Here's how the part is built. I have some questions about the finished solid (model axes, mm). Face numbers are marked on the shaded views. A direction names the side the tool comes from. Coordinates: 2 decimals unless noted, no trailing zeros.
Item 1: I'm going to push flat-ended pins straight in: pin 1 Ø8 at (x, z) = (43.5, 32.5) entering from -Y; pin 2 Ø15 at (x, z) = (70, 6) entering from -Y; pin 3 Ø21.5 at (x, z) = (-11.5, 15) entering from -Y. Where does each tip first touch, or does it pass through?
Item 2: If I drill on line 1 (X direction, y = -20.5, z = -4.5); line 2 (X direction, y = -19.5, z = 1); line 3 (Y direction, x = 37.5, z = -2), over which ranges is the centre line in solid material (lowest first)?
Item 3: We'd pull the mould along Z, two halves only. Please class the marked faces 1, 2 and 3: +Z half, -Z half, draft (parallel to the pull), parting line (faces both ways), or undercut.
Item 4: For the marked faces 4 and 5, which set-ups out of +Z, -Z, +X, -X, +Y, -Y let a thin tool reach every point of the face, with its end or its side?
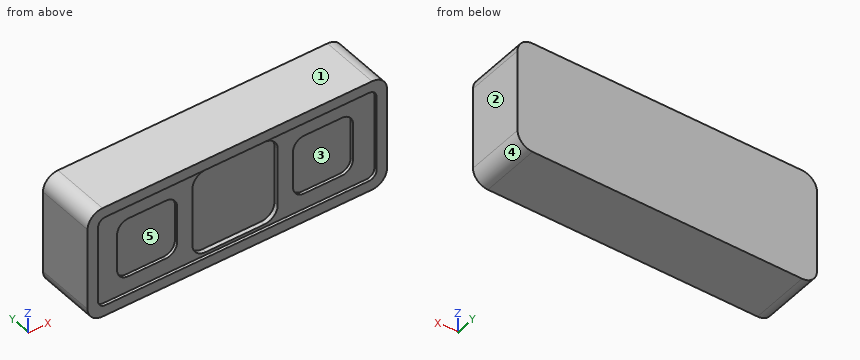
from build123d import *

# Parameters (mm, degrees)
F0_R     = 32.385
F0_R_2   = 20.32
F1_DEPTH = 25.4
F3_DEPTH = 2.54
F5_DEPTH = 3.81
F5_TAPER = -0.25
F7_DEPTH = 2.54
F7_TAPER = -0.25


with BuildPart() as f1:
    # F0 (on Front) → F1 (new body, symmetric)
    with BuildSketch(Plane.XZ):
        with BuildLine():
            Line((114.3, 47.625), (-114.3, 47.625))
            ThreePointArc((-114.3, 47.625), (-123.2802561211, 43.9052561211), (-127, 34.925))
            Line((-127, 34.925), (-127, -34.925))
            ThreePointArc((-127, -34.925), (-123.2802561211, -43.9052561211), (-114.3, -47.625))
            Line((-114.3, -47.625), (114.3, -47.625))
            ThreePointArc((114.3, -47.625), (123.2802561211, -43.9052561211), (127, -34.925))
            Line((127, -34.925), (127, 34.925))
            ThreePointArc((127, 34.925), (123.2802561211, 43.9052561211), (114.3, 47.625))
        make_face()
        Circle(F0_R, mode=Mode.SUBTRACT)
        with Locations((-74.5998, 0)):
            Circle(F0_R_2, mode=Mode.SUBTRACT)
        with Locations((74.5998, 0)):
            Circle(F0_R_2, mode=Mode.SUBTRACT)
        with Locations((74.5998, 0)):
            Circle(F0_R_2)
        Circle(F0_R)
        with Locations((-74.5998, 0)):
            Circle(F0_R_2)
    extrude(amount=F1_DEPTH, both=True)

    # F2 (on face) → F3 (cut)
    with BuildSketch(Plane.XZ.offset(25.4)):
        with BuildLine():
            Line((-111.76, -38.735), (111.76, -38.735))
            ThreePointArc((111.76, -38.735), (116.2501280605, -36.8751280605), (118.11, -32.385))
            Line((118.11, -32.385), (118.11, 32.385))
            ThreePointArc((118.11, 32.385), (116.2501280605, 36.8751280605), (111.76, 38.735))
            Line((111.76, 38.735), (-111.76, 38.735))
            ThreePointArc((-111.76, 38.735), (-116.2501280605, 36.8751280605), (-118.11, 32.385))
            Line((-118.11, 32.385), (-118.11, -32.385))
            ThreePointArc((-118.11, -32.385), (-116.2501280605, -36.8751280605), (-111.76, -38.735))
        make_face()
    extrude(amount=-F3_DEPTH, mode=Mode.SUBTRACT)

    # F4 (on face) → F5 (cut)
    with BuildSketch(Plane.XZ.offset(22.86)):
        with BuildLine():
            Line((24.765, 36.195), (-24.765, 36.195))
            ThreePointArc((-24.765, 36.195), (-32.847230509, 32.847230509), (-36.195, 24.765))
            Line((-36.195, 24.765), (-36.195, -24.765))
            ThreePointArc((-36.195, -24.765), (-32.847230509, -32.847230509), (-24.765, -36.195))
            Line((-24.765, -36.195), (24.765, -36.195))
            ThreePointArc((24.765, -36.195), (32.847230509, -32.847230509), (36.195, -24.765))
            Line((36.195, -24.765), (36.195, 24.765))
            ThreePointArc((36.195, 24.765), (32.847230509, 32.847230509), (24.765, 36.195))
        make_face()
    extrude(amount=-F5_DEPTH, taper=F5_TAPER, mode=Mode.SUBTRACT)

    # F6 (on face) → F7 (cut)
    with BuildSketch(Plane.XZ.offset(22.86)):
        with BuildLine():
            Line((-58.7248, 25.4), (-90.4748, 25.4))
            ThreePointArc((-90.4748, 25.4), (-97.2099920908, 22.6101920908), (-99.9998, 15.875))
            Line((-99.9998, 15.875), (-99.9998, -15.875))
            ThreePointArc((-99.9998, -15.875), (-97.2099920908, -22.6101920908), (-90.4748, -25.4))
            Line((-90.4748, -25.4), (-58.7248, -25.4))
            ThreePointArc((-58.7248, -25.4), (-51.9896079092, -22.6101920908), (-49.1998, -15.875))
            Line((-49.1998, -15.875), (-49.1998, 15.875))
            ThreePointArc((-49.1998, 15.875), (-51.9896079092, 22.6101920908), (-58.7248, 25.4))
        make_face()
        with BuildLine():
            ThreePointArc((99.9998, 15.875), (97.2099920908, 22.6101920908), (90.4748, 25.4))
            Line((90.4748, 25.4), (58.7248, 25.4))
            ThreePointArc((58.7248, 25.4), (51.9896079092, 22.6101920908), (49.1998, 15.875))
            Line((49.1998, 15.875), (49.1998, -15.875))
            ThreePointArc((49.1998, -15.875), (51.9896079092, -22.6101920908), (58.7248, -25.4))
            Line((58.7248, -25.4), (90.4748, -25.4))
            ThreePointArc((90.4748, -25.4), (97.2099920908, -22.6101920908), (99.9998, -15.875))
            Line((99.9998, -15.875), (99.9998, 15.875))
        make_face()
    extrude(amount=-F7_DEPTH, taper=F7_TAPER, mode=Mode.SUBTRACT)


solid = f1.part
Answer list:
1. pin 1: stops at y = -22.86
1. pin 2: stops at y = -20.32
1. pin 3: stops at y = -19.05
2. line 1: x = -127 to -100.01, -49.19 to -36.21, 36.21 to 49.19, 100.01 to 127
2. line 2: x = -127 to -36.21, 36.21 to 127
2. line 3: y = -22.86 to 25.4
3. face 1: +Z half
3. face 2: draft
3. face 3: undercut
4. face 4: -Z, +X, +Y, -Y
4. face 5: -Y
